Build history of the part. All positions in model axes, mm. A direction names the side the tool comes from. Round coordinates to 2 decimals unless told otherwise and drop trailing zeros. Write each loop counter-clockwise with the first axis right and the second up, starting at its lowest first coordinate (ties: lowest second). Pieces come first, ordered by that corner, then holes. Notation, with made-up numbers: M 2,23 L 38,23 A32 ccw 38,55 Z; hole C 80.5,17 d9. An arc over 180 degrees is marked long. Write item = value, one per line.
from build123d import *

# Parameters (mm, degrees)
SKETCH1_W                                  = 48
SKETCH1_H                                  = 50
BOSS_EXTRUDE1_DEPTH                        = 10
SKETCH2_W                                  = 20
SKETCH2_H                                  = 20
CUT_EXTRUDE1_DEPTH                         = 10
CBORE_FOR_M6_CHEESE_HEAD_SCREW1_AT_2_COUNT = 2
CBORE_FOR_M6_CHEESE_HEAD_SCREW1_AT_2_PITCH = 22
CBORE_FOR_M6_CHEESE_HEAD_SCREW1_AT_3_COUNT = 2
CBORE_FOR_M6_CHEESE_HEAD_SCREW1_AT_3_PITCH = 38.832975678
CBORE_FOR_M6_CHEESE_HEAD_SCREW1_AT_4_COUNT = 2
CBORE_FOR_M6_CHEESE_HEAD_SCREW1_AT_4_PITCH = 32


with BuildPart() as part:
    # Sketch1 → Boss-Extrude1 (new body)
    with BuildSketch(Plane(origin=(0, 0, 0), x_dir=(1, 0, 0), z_dir=(0, 1, 0))):
        Rectangle(SKETCH1_W, SKETCH1_H)
    extrude(amount=BOSS_EXTRUDE1_DEPTH)

    # Sketch2 → Cut-Extrude1 (cut)
    with BuildSketch(Plane(origin=(0, 10, 0), x_dir=(1, 0, 0), z_dir=(0, 1, 0))):
        with Locations((0, 25)):
            Rectangle(SKETCH2_W, SKETCH2_H)
    extrude(amount=-CUT_EXTRUDE1_DEPTH, mode=Mode.SUBTRACT)

    # Sketch4 → CBORE for M6 Cheese Head Screw1 (revolve, cut)
    with BuildSketch(Plane(origin=(-16, 10, -7), x_dir=(0, 0, 1), z_dir=(1, 0, 0))):
        Polygon((0, 0), (0, 11.982840043), (3.3, 10), (3.3, 3.9), (5.5, 3.9), (5.5, 0.025), (5.525, 0), align=None)
    cbore_for_m6_cheese_head_screw1 = revolve(axis=Axis((-16, 16.35, -7), (0, -1, 0)), mode=Mode.SUBTRACT)

    # CBORE for M6 Cheese Head Screw1 at 2: CBORE for M6 Cheese Head Screw1 ×2
    with Locations(*[(0, 0, i * CBORE_FOR_M6_CHEESE_HEAD_SCREW1_AT_2_PITCH) for i in range(1, CBORE_FOR_M6_CHEESE_HEAD_SCREW1_AT_2_COUNT)]):
        add(cbore_for_m6_cheese_head_screw1, mode=Mode.SUBTRACT)

    # CBORE for M6 Cheese Head Screw1 at 3: CBORE for M6 Cheese Head Screw1 ×2
    with Locations(*[Vector(0.8240419241993677, 0, 0.5665288228870652) * (i * CBORE_FOR_M6_CHEESE_HEAD_SCREW1_AT_3_PITCH) for i in range(1, CBORE_FOR_M6_CHEESE_HEAD_SCREW1_AT_3_COUNT)]):
        add(cbore_for_m6_cheese_head_screw1, mode=Mode.SUBTRACT)

    # CBORE for M6 Cheese Head Screw1 at 4: CBORE for M6 Cheese Head Screw1 ×2
    with Locations(*[(i * CBORE_FOR_M6_CHEESE_HEAD_SCREW1_AT_4_PITCH, 0, 0) for i in range(1, CBORE_FOR_M6_CHEESE_HEAD_SCREW1_AT_4_COUNT)]):
        add(cbore_for_m6_cheese_head_screw1, mode=Mode.SUBTRACT)


solid = part.part
1. Mould opens along X. For faces 4 (the face through (0, 5, -15)), 5 (the face through (17, 5, -25)), 6 (the face through (-24, 5, 0)) say: pulls with the +X half, pulls with the -X half, needs draft (parallel to the pull), parting line crosses it, or undercut.
Responses:
face_4 = undercut
face_5 = needs draft
face_6 = pulls with the -X half
2. Tool access for faces 1 (the face through (10, 5, -20)), 2 (the face through (-11.1, 8.1, -4.5)), 3 (the face through (0, 5, 25)): list every direction of +Z, -Z, +X, -X, +Y, -Y with a clear straight run to the whole face (end or side of a thin tool).
Responses:
face_1 = -Z, +Y, -Y
face_2 = +Y
face_3 = +Z, +X, -X, +Y, -Y
3. Band-saw the part on A-A (z = -18.5). List the corners of the cut face in (x, y).
Responses:
outline = M -24,0 L -10,0 L -10,10 L -24,10 Z; M 10,0 L 24,0 L 24,10 L 10,10 Z
4. Probe probe 1 along X at (y, z) = (6.9, 15); probe 2 along Z at (x, y) = (-16, 8.9); probe 3 along X at (y, z) = (4.5, 15). List the from-to ranges inside material, lowest first.
Responses:
probe_1 = -24 to -21.5, -10.5 to 10.5, 21.5 to 24
probe_2 = -25 to -12.5, -1.5 to 9.5, 20.5 to 25
probe_3 = -24 to -19.3, -12.7 to 12.7, 19.3 to 24
5. Flat gauge pins, fed straight in: pin 1 (1.5 mm diameter, centred on x = -17.5, z = 12.5, fed in from +Y); pin 2 (3 mm diameter, centred on x = -2.5, y = 6, fed in from -Z); pin 3 (5.5 mm diameter, centred on x = 16, z = 15, fed in from +Y). Where does each tip first touch, or does it go through?
Responses:
pin_1 = 6.1
pin_2 = -15
pin_3 = through
6. Band-saw the part on D-D (z = 15). List the corners of the cut face in (x, y) (3 decimals), plus the area to 3 significant figures.
Responses:
outline = M -24,0 L -19.3,0 L -19.3,6.1 L -21.5,6.1 L -21.5,9.975 L -21.525,10 L -24,10 Z; M -12.7,0 L 12.7,0 L 12.7,6.1 L 10.5,6.1 L 10.5,9.975 L 10.475,10 L -10.475,10 L -10.5,9.975 L -10.5,6.1 L -12.7,6.1 Z; M 19.3,0 L 24,0 L 24,10 L 21.525,10 L 21.5,9.975 L 21.5,6.1 L 19.3,6.1 Z
area = 314 mm²
7. Band-saw the part on B-B (x = 16). List the corners of the cut face in (y, z) (3 decimals).
Responses:
outline = M 0,-25 L 10,-25 L 10,-12.525 L 9.975,-12.5 L 6.1,-12.5 L 6.1,-10.3 L 0,-10.3 Z; M 0,-3.7 L 6.1,-3.7 L 6.1,-1.5 L 9.975,-1.5 L 10,-1.475 L 10,9.475 L 9.975,9.5 L 6.1,9.5 L 6.1,11.7 L 0,11.7 Z; M 0,18.3 L 6.1,18.3 L 6.1,20.5 L 9.975,20.5 L 10,20.525 L 10,25 L 0,25 Z
8. Band-saw the part on C-C (y = 6.75). List the corners of the cut face in (x, z), plus the area to 3 significant figures.
Responses:
outline = M -24,-25 L -10,-25 L -10,-15 L 10,-15 L 10,-25 L 24,-25 L 24,25 L -24,25 Z; hole C -16,-7 d11; hole C -16,15 d11; hole C 16,-7 d11; hole C 16,15 d11
area = 1,820 mm²
